Input: part model. Units: mm. Frame: model coordinates. Face numbers are marked on the shaded views. A direction names the side the tool comes from. Give positions to 0.01 mm unless a question says otherwise; leave off trailing zeros. Loops run counter-clockwise (first coordinate to the right, second up) from the corner with the lowest first, then second, coordinate; pieces in that order, holes last. Notation, with made-up numbers: M 37,59.25 L 45,59.25 A24 ccw 45,78.25 Z; hole C -2.75,54 d11. An arc over 180 degrees is marked long. One line per item, written item: value. Start each with the question number.
(1) Section A-A on y = -8. Output: boundary loops of the cut face in (x, z), plus the area to 3 significant figures.
(2) Ray query, line 1 along Z through (x, y) = (-66, -16). Return the intervals inside material, ascending. Write a range as from..to.
(3) Access query for the marked faces 1 and 2. Directions: +Z, -Z, +X, -X, +Y, -Y. A direction counts if a zero-diameter tool reaches every point of the face in a straight line with its end or side. Return the directions, or none.
(4) Section B-B on z = 8.5. Output: boundary loops of the cut face in (x, y).
(5) Pin query (flat end, axial travel): P1, Ø16.5, axis at x = -35.5, y = -8.5, coming from the -Z side; P2, Ø3.5, axis at y = -25, z = 10, coming from the +X side. Return the tip coordinate at first contact, or that it passes through.
(6) Section C-C on x = -66. Output: boundary loops of the cut face in (y, z).
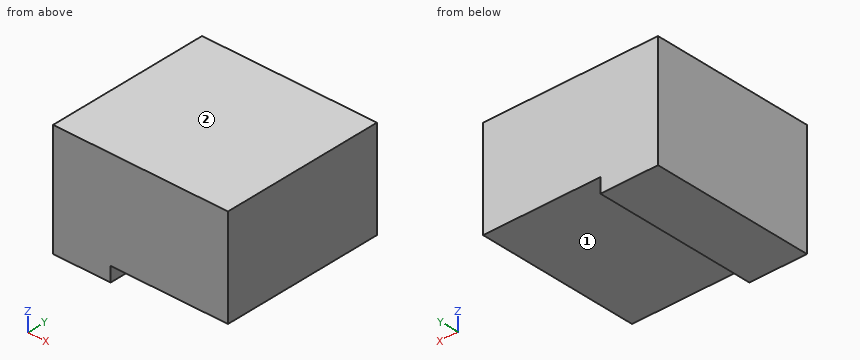
```python
from build123d import *

# Parameters (mm, degrees)
F1_DEPTH      = 50.8
F1_DEPTH_BACK = 25.4


with BuildPart() as f1:
    # F0 (on Front) → F1 (new body, two sides)
    with BuildSketch(Plane.XZ) as f1_sk:
        Polygon((-19.007457, 58.110539), (-100.5354, 58.110539), (-100.5354, 5.079421), (-73.713064, 5.079421), (-73.713064, 11.915244), (-19.007457, 11.915244), align=None)
    extrude(amount=F1_DEPTH)
    extrude(f1_sk.sketch, amount=-F1_DEPTH_BACK)


solid = f1.part
```
Output values:
1. outline: M -100.54,5.08 L -73.71,5.08 L -73.71,11.92 L -19.01,11.92 L -19.01,58.11 L -100.54,58.11 Z
1. area: 3,950 mm²
2. line 1: z = 11.92..58.11
3. face 1: -Z, +X, +Y, -Y
3. face 2: +Z, +X, -X, +Y, -Y
4. outline: M -100.54,-50.8 L -73.71,-50.8 L -73.71,25.4 L -100.54,25.4 Z
5. P1: stops at z = 11.92
5. P2: stops at x = -73.71
6. outline: M -50.8,11.92 L 25.4,11.92 L 25.4,58.11 L -50.8,58.11 Z
